Can you work these out from the model? Positions are in its coordinate system, mm. Give positions to 0.01 mm unless a question says otherwise; leave off trailing zeros. Order: outer loops, then holes, each group sorted by start corner. A loop starts at its lowest first (then second) coordinate and runs counter-clockwise, first axis right, second up. Notation, with made-up numbers: (63, 70) - (78, 70) arc R36 ccw to (78, 108) - close; hole circle Ø11 at (-1.75, 40.5). An arc over 180 degrees is marked (long way). One line per question, with ' | ' between items.
Autodesk Inventor part; units mm, degrees
ref_plane "YZ Plane" through (0, 0, 0) normal (1, 0, 0) x (0, 1, 0)
ref_plane "XZ Plane" through (0, 0, 0) normal (0, 1, 0) x (-1, 0, 0)
ref_plane "XY Plane" through (0, 0, 0) normal (0, 0, 1) x (1, 0, 0)
sketch "スケッチ1" plane through (0, 0, 0) normal (0, 0, 1) x (1, 0, 0)
  circle A0 centre (0, 0) radius 57
  circle A1 centre (0, 0) radius 44.5
  dimension "d0" = 114
  dimension "d1" = 89
extrude "押し出し1" add sketch "スケッチ1" along normal blind 8.2
sketch "スケッチ2" plane through (0, 0, 8.2) normal (0, 0, 1) x (1, 0, 0)
  point P0 (0, 0)
  point P1 (0, -50.75)
  point P2 (50.75, 0)
  point P3 (0, 50.75)
  point P4 (-50.75, 0)
  dimension "d4" = 50.75
  dimension "d7" = 360
hole "穴1" at (0, -50.75, 8.2) at (50.75, 0, 8.2) at (0, 50.75, 8.2) at (-50.75, 0, 8.2) direction (0, 0, -1) diameter 4.4 end through all countersink diameter 10 countersink angle 90
fillet "フィレット1" radius 0.5 4 edges at (-57, 0, 8.2) (-44.5, 0, 8.2) (-57, 0, 0) (-44.5, 0, 0)
properties part number "TurnTable140_Inner" material "鋼、合金"
(1) Will these pins go through, and if not, where does the flat tip stop? pin 1 (5 mm diameter, centred on x = 0, y = 50.75, fed in from +Z); pin 2 (4 mm diameter, centred on y = -34.5, z = 2.5, fed in from -X); pin 3 (5.5 mm diameter, centred on x = 50.75, y = 0, fed in from +Z); pin 4 (12 mm diameter, centred on x = -32, y = 27.5, fed in from +Z).
Answer below:
pin 1: z = 5.7 | pin 2: x = -46.83 | pin 3: z = 5.95 | pin 4: z = 8.2
(2) If we mould it in two halves opening along X, with no side actions, what happens to faces 1 (the face through (-17, 42, 0)), 2 (the face through (-0.097, 52.948, 2.662)), 3 (the face through (52.654, 21.831, 4.05))? For each: released by +X, released by -X, zero draft, split by the parting line, or undercut.
Answer below:
face 1: zero draft | face 2: undercut | face 3: split by the parting line
(3) Imagine slicing it at A-A (y = 0). List the corners of the cut face in (x, z) for me.
Answer below:
outline: (-57, 0.5) arc R0.5 ccw to (-56.5, 0) - (-52.95, 0) - (-52.95, 5.4) - (-55.75, 8.2) - (-56.5, 8.2) arc R0.5 ccw to (-57, 7.7) - close; (-48.55, 0) - (-45, 0) arc R0.5 ccw to (-44.5, 0.5) - (-44.5, 7.7) arc R0.5 ccw to (-45, 8.2) - (-45.75, 8.2) - (-48.55, 5.4) - close; (44.5, 0.5) arc R0.5 ccw to (45, 0) - (48.55, 0) - (48.55, 5.4) - (45.75, 8.2) - (45, 8.2) arc R0.5 ccw to (44.5, 7.7) - close; (52.95, 0) - (56.5, 0) arc R0.5 ccw to (57, 0.5) - (57, 7.7) arc R0.5 ccw to (56.5, 8.2) - (55.75, 8.2) - (52.95, 5.4) - close
(4) If I drill on line 1 (Y direction, x = 0, z = 1.85); line 2 (Y direction, x = -1, z = 6.5); line 3 (Y direction, x = -19, z = 6), over which ranges is the centre line in solid material (lowest first)?
Answer below:
line 1: -57 to -52.95, -48.55 to -44.5, 44.5 to 48.55, 52.95 to 57 | line 2: -56.99 to -53.89, -47.61 to -44.49, 44.49 to 47.61, 53.89 to 56.99 | line 3: -53.74 to -40.24, 40.24 to 53.74
(5) Imagine slicing it at C-C (z = 2). List the corners of the cut face in (x, y) for me, and give its area (3 significant figures).
Answer below:
outline: circle Ø114 at (0, 0); hole circle Ø4.4 at (-50.75, 0); hole circle Ø89 at (0, 0); hole circle Ø4.4 at (0, -50.75); hole circle Ø4.4 at (0, 50.75); hole circle Ø4.4 at (50.75, 0) | area: 3,930 mm^2
